Could you check a few things on this model? Use its own coordinates, in mm. Give positions to 0.01 mm unless a question says otherwise; leave off trailing zeros.
1. Thinking about a two-plate mould opening in Z: for faces 1 (the flat face through (-1, -2000, 11)), 2 (the flat face through (0, -986, -28)), which applies, +Z half, -Z half, draft (parallel to the pull), parting line (faces both ways), or undercut?
2. Imagine slicing it at A-A (y = -971). Count the separate pieces of the cut face and the enclosed holes in it, plus the area to 3 significant figures.
3. I need wall thicknesses on line 1 along X through (y, z) = (-1684, -28.5); line 2 along Z through (x, y) = (-36, -1428); line 3 along X through (y, z) = (-405.5, -36.25). Which ranges of each line are inside material? Lowest first, please.
4. For P1, Ø1, axis at y = -932.5, z = 5.5, coming from the +X side; P2, Ø3, axis at y = -963, z = -42.5, coming from the +X side; P3, Ø5, axis at y = -1248, z = -22, coming from the -X side, each with a flat end and sliding along its axis, tell me the tip position at first contact or that it passes through.
```python
from build123d import *

# Parameters (mm, degrees)
F1_DEPTH = 2000


with BuildPart() as f1:
    # F0 (on Front) → F1 (new body)
    with BuildSketch(Plane.XZ):
        with BuildLine():
            ThreePointArc((0, -7.5), (-5.303301, -5.303301), (-7.5, 0))
            Line((-7.5, 0), (-12, 0))
            Line((-12, 0), (-12, -9.5))
            Line((-12, -9.5), (-28, -25.5))
            Line((-28, -25.5), (-28, 0))
            Line((-28, 0), (-33.25, 0))
            ThreePointArc((-33.25, 0), (-36.25, -3), (-39.25, 0))
            Line((-39.25, 0), (-44.5, 0))
            Line((-44.5, 0), (-44.5, -9.5))
            Line((-44.5, -9.5), (-45, -9.5))
            Line((-45, -9.5), (-45, -17))
            Line((-45, -17), (-44.5, -17))
            Line((-44.5, -17), (-44.5, -17.5))
            Line((-44.5, -17.5), (-39, -17.5))
            Line((-39, -17.5), (-39, -12.5))
            Line((-39, -12.5), (-32, -12.5))
            Line((-32, -12.5), (-32, -29.5))
            Line((-32, -29.5), (-36, -33.5))
            Line((-36, -33.5), (-39, -33.5))
            Line((-39, -33.5), (-39, -27.5))
            Line((-39, -27.5), (-44.5, -27.5))
            Line((-44.5, -27.5), (-44.5, -28))
            Line((-44.5, -28), (-45, -28))
            Line((-45, -28), (-45, -40))
            ThreePointArc((-45, -40), (-43.535534, -43.535534), (-40, -45))
            Line((-40, -45), (-28, -45))
            Line((-28, -45), (-28, -44.5))
            Line((-28, -44.5), (-27.5, -44.5))
            Line((-27.5, -44.5), (-27.5, -39))
            Line((-27.5, -39), (-33.5, -39))
            Line((-33.5, -39), (-33.5, -36))
            Line((-33.5, -36), (-29.5, -32))
            Line((-29.5, -32), (-12.5, -32))
            Line((-12.5, -32), (-12.5, -39))
            Line((-12.5, -39), (-17.5, -39))
            Line((-17.5, -39), (-17.5, -44.5))
            Line((-17.5, -44.5), (-17, -44.5))
            Line((-17, -44.5), (-17, -45))
            Line((-17, -45), (-9.5, -45))
            Line((-9.5, -45), (-9.5, -44.5))
            Line((-9.5, -44.5), (0, -44.5))
            Line((0, -44.5), (0, -39.25))
            ThreePointArc((0, -39.25), (-3, -36.25), (0, -33.25))
            Line((0, -33.25), (0, -28))
            Line((0, -28), (-25.5, -28))
            Line((-25.5, -28), (-9.5, -12))
            Line((-9.5, -12), (0, -12))
            Line((0, -12), (0, -7.5))
        make_face()
        with BuildLine():
            Line((0, 39.25), (0, 44.5))
            Line((0, 44.5), (-9.5, 44.5))
            Line((-9.5, 44.5), (-9.5, 45))
            Line((-9.5, 45), (-17, 45))
            Line((-17, 45), (-17, 44.5))
            Line((-17, 44.5), (-17.5, 44.5))
            Line((-17.5, 44.5), (-17.5, 39))
            Line((-17.5, 39), (-12.5, 39))
            Line((-12.5, 39), (-12.5, 32))
            Line((-12.5, 32), (-29.5, 32))
            Line((-29.5, 32), (-33.5, 36))
            Line((-33.5, 36), (-33.5, 39))
            Line((-33.5, 39), (-27.5, 39))
            Line((-27.5, 39), (-27.5, 44.5))
            Line((-27.5, 44.5), (-28, 44.5))
            Line((-28, 44.5), (-28, 45))
            Line((-28, 45), (-40, 45))
            ThreePointArc((-40, 45), (-43.535534, 43.535534), (-45, 40))
            Line((-45, 40), (-45, 28))
            Line((-45, 28), (-44.5, 28))
            Line((-44.5, 28), (-44.5, 27.5))
            Line((-44.5, 27.5), (-39, 27.5))
            Line((-39, 27.5), (-39, 33.5))
            Line((-39, 33.5), (-36, 33.5))
            Line((-36, 33.5), (-32, 29.5))
            Line((-32, 29.5), (-32, 12.5))
            Line((-32, 12.5), (-39, 12.5))
            Line((-39, 12.5), (-39, 17.5))
            Line((-39, 17.5), (-44.5, 17.5))
            Line((-44.5, 17.5), (-44.5, 17))
            Line((-44.5, 17), (-45, 17))
            Line((-45, 17), (-45, 9.5))
            Line((-45, 9.5), (-44.5, 9.5))
            Line((-44.5, 9.5), (-44.5, 0))
            Line((-44.5, 0), (-39.25, 0))
            ThreePointArc((-39.25, 0), (-36.25, 3), (-33.25, 0))
            Line((-33.25, 0), (-28, 0))
            Line((-28, 0), (-28, 25.5))
            Line((-28, 25.5), (-12, 9.5))
            Line((-12, 9.5), (-12, 0))
            Line((-12, 0), (-7.5, 0))
            ThreePointArc((-7.5, 0), (-5.303301, 5.303301), (0, 7.5))
            Line((0, 7.5), (0, 12))
            Line((0, 12), (-9.5, 12))
            Line((-9.5, 12), (-25.5, 28))
            Line((-25.5, 28), (0, 28))
            Line((0, 28), (0, 33.25))
            ThreePointArc((0, 33.25), (-3, 36.25), (0, 39.25))
        make_face()
        with BuildLine():
            Line((40, 45), (28, 45))
            Line((28, 45), (28, 44.5))
            Line((28, 44.5), (27.5, 44.5))
            Line((27.5, 44.5), (27.5, 39))
            Line((27.5, 39), (33.5, 39))
            Line((33.5, 39), (33.5, 36))
            Line((33.5, 36), (29.5, 32))
            Line((29.5, 32), (12.5, 32))
            Line((12.5, 32), (12.5, 39))
            Line((12.5, 39), (17.5, 39))
            Line((17.5, 39), (17.5, 44.5))
            Line((17.5, 44.5), (17, 44.5))
            Line((17, 44.5), (17, 45))
            Line((17, 45), (9.5, 45))
            Line((9.5, 45), (9.5, 44.5))
            Line((9.5, 44.5), (0, 44.5))
            Line((0, 44.5), (0, 39.25))
            ThreePointArc((0, 39.25), (3, 36.25), (0, 33.25))
            Line((0, 33.25), (0, 28))
            Line((0, 28), (25.5, 28))
            Line((25.5, 28), (9.5, 12))
            Line((9.5, 12), (0, 12))
            Line((0, 12), (0, 7.5))
            ThreePointArc((0, 7.5), (5.303301, 5.303301), (7.5, 0))
            Line((7.5, 0), (12, 0))
            Line((12, 0), (12, 9.5))
            Line((12, 9.5), (28, 25.5))
            Line((28, 25.5), (28, 0))
            Line((28, 0), (33.25, 0))
            ThreePointArc((33.25, 0), (36.25, 3), (39.25, 0))
            Line((39.25, 0), (44.5, 0))
            Line((44.5, 0), (44.5, 9.5))
            Line((44.5, 9.5), (45, 9.5))
            Line((45, 9.5), (45, 17))
            Line((45, 17), (44.5, 17))
            Line((44.5, 17), (44.5, 17.5))
            Line((44.5, 17.5), (39, 17.5))
            Line((39, 17.5), (39, 12.5))
            Line((39, 12.5), (32, 12.5))
            Line((32, 12.5), (32, 29.5))
            Line((32, 29.5), (36, 33.5))
            Line((36, 33.5), (39, 33.5))
            Line((39, 33.5), (39, 27.5))
            Line((39, 27.5), (44.5, 27.5))
            Line((44.5, 27.5), (44.5, 28))
            Line((44.5, 28), (45, 28))
            Line((45, 28), (45, 40))
            ThreePointArc((45, 40), (43.535534, 43.535534), (40, 45))
        make_face()
        with BuildLine():
            Line((44.5, -9.5), (44.5, 0))
            Line((44.5, 0), (39.25, 0))
            ThreePointArc((39.25, 0), (36.25, -3), (33.25, 0))
            Line((33.25, 0), (28, 0))
            Line((28, 0), (28, -25.5))
            Line((28, -25.5), (12, -9.5))
            Line((12, -9.5), (12, 0))
            Line((12, 0), (7.5, 0))
            ThreePointArc((7.5, 0), (5.303301, -5.303301), (0, -7.5))
            Line((0, -7.5), (0, -12))
            Line((0, -12), (9.5, -12))
            Line((9.5, -12), (25.5, -28))
            Line((25.5, -28), (0, -28))
            Line((0, -28), (0, -33.25))
            ThreePointArc((0, -33.25), (3, -36.25), (0, -39.25))
            Line((0, -39.25), (0, -44.5))
            Line((0, -44.5), (9.5, -44.5))
            Line((9.5, -44.5), (9.5, -45))
            Line((9.5, -45), (17, -45))
            Line((17, -45), (17, -44.5))
            Line((17, -44.5), (17.5, -44.5))
            Line((17.5, -44.5), (17.5, -39))
            Line((17.5, -39), (12.5, -39))
            Line((12.5, -39), (12.5, -32))
            Line((12.5, -32), (29.5, -32))
            Line((29.5, -32), (33.5, -36))
            Line((33.5, -36), (33.5, -39))
            Line((33.5, -39), (27.5, -39))
            Line((27.5, -39), (27.5, -44.5))
            Line((27.5, -44.5), (28, -44.5))
            Line((28, -44.5), (28, -45))
            Line((28, -45), (40, -45))
            ThreePointArc((40, -45), (43.535534, -43.535534), (45, -40))
            Line((45, -40), (45, -28))
            Line((45, -28), (44.5, -28))
            Line((44.5, -28), (44.5, -27.5))
            Line((44.5, -27.5), (39, -27.5))
            Line((39, -27.5), (39, -33.5))
            Line((39, -33.5), (36, -33.5))
            Line((36, -33.5), (32, -29.5))
            Line((32, -29.5), (32, -12.5))
            Line((32, -12.5), (39, -12.5))
            Line((39, -12.5), (39, -17.5))
            Line((39, -17.5), (44.5, -17.5))
            Line((44.5, -17.5), (44.5, -17))
            Line((44.5, -17), (45, -17))
            Line((45, -17), (45, -9.5))
            Line((45, -9.5), (44.5, -9.5))
        make_face()
    extrude(amount=F1_DEPTH)


solid = f1.part
```
Derived:
1. face 1: draft
1. face 2: undercut
2. separate pieces: 1
2. enclosed holes: 9
2. area: 3,910 mm2
3. line 1: x = -45 to -39, -32 to 32, 39 to 45
3. line 2: z = -45 to -33.5, -12.5 to -2.99, 2.99 to 12.5, 33.5 to 45
3. line 3: x = -45 to -33.5, -12.5 to -3, 3 to 12.5, 33.5 to 45
4. P1: stops at x = 44.5
4. P2: stops at x = 44.9
4. P3: stops at x = -32
